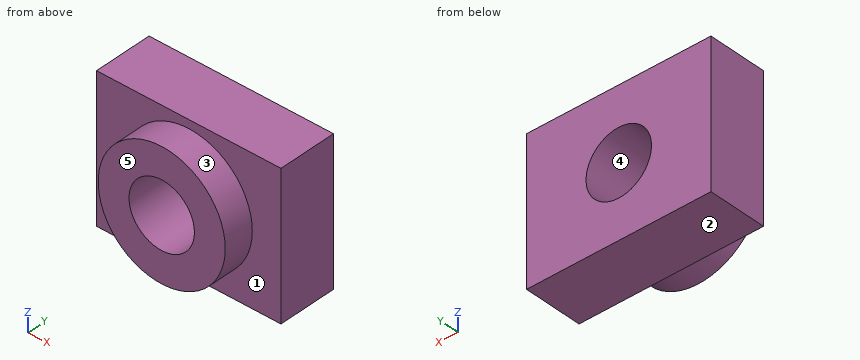
from build123d import *

# Parameters (mm, degrees)
F0_R          = 35.778337
F0_R_2        = 18.424751
F1_DEPTH      = 25
F1_DEPTH_BACK = 25
F0_W          = 103.87025
F0_H          = 80.97905
F2_DEPTH      = 8
F2_DEPTH_BACK = 25


with BuildPart() as f1:
    # F0 (on Front) → F1 (new body, two sides)
    with BuildSketch(Plane.XZ) as f1_sk:
        Circle(F0_R)
        Circle(F0_R_2, mode=Mode.SUBTRACT)
    extrude(amount=F1_DEPTH)
    extrude(f1_sk.sketch, amount=-F1_DEPTH_BACK)

    # F0 (on Front) → F2 (join, two sides)
    with BuildSketch(Plane.XZ) as f2_sk:
        Rectangle(F0_W, F0_H)
        Circle(F0_R, mode=Mode.SUBTRACT)
    extrude(amount=F2_DEPTH)
    extrude(f2_sk.sketch, amount=-F2_DEPTH_BACK)


solid = f1.part
The listing builds one solid part. Answer for the finished solid, in the listing's coordinates (mm). Face numbers are marked on the shaded views. A direction names the side the tool comes from. Round coordinates to 2 decimals unless told otherwise and drop trailing zeros. Write each loop counter-clockwise with the first axis right and the second up, starting at its lowest first coordinate (ties: lowest second). Pieces come first, ordered by that corner, then holes. Notation, with made-up numbers: (61, 3.25) - (82, 3.25) arc R22 cw to (82, 27.25) - close; hole circle Ø8 at (34, 66.5). An arc over 180 degrees is marked (long way). Use one line per item in the form item = value. Start each with the question number.
Item 1: A cutting plane is placed at A-A (z = 0). Write down the section's boundary in (x, y).
Item 2: Determine the mould class of the marked faces 3, 4 and 5 for opening direction Z: +Z half, -Z half, draft (parallel to the pull), parting line (faces both ways), or undercut.
Item 3: Find the intervals of material crossed by line 1 (Z direction, x = 0, y = -12); line 2 (Z direction, x = 0, y = 7); line 3 (Y direction, x = -33.5, z = 29), in increasing order. Write a range as [from, to].
Item 4: A cutting plane is placed at B-B (x = 0). Write down the section's boundary in (y, z), plus the area to 3 significant figures.
Item 5: A cutting plane is placed at C-C (y = -5). Write down the section's boundary in (x, z), plus the area to 3 significant figures.
Item 6: Flat-ended cylindrical pins translate along their axes: pin 1 Ø4 at (y, z) = (-19, 15) entering from +X; pin 2 Ø8 at (y, z) = (-13.5, 27.5) entering from -X; pin 3 Ø3 at (x, z) = (-11, 14.5) entering from +Y; pin 4 Ø2 at (x, z) = (-37, -4.5) entering from -Y. Find the tip coordinate at first contact, or state that the pin passes through.
Item 7: A cutting plane is placed at D-D (z = -26). Write down the section's boundary in (x, y), plus the area to 3 significant figures.
Item 8: A tool of negligible diameter and unlimited length cuts with its end or side. For the marked faces 1 and 2, from which of +Z, -Z, +X, -X, +Y, -Y can it reach the whole face along a straight path? Write none if from no direction.
The answers:
q1.outline = (-51.94, -8) - (-35.78, -8) - (-35.78, -25) - (-18.42, -25) - (-18.42, 25) - (-51.94, 25) - close; (18.42, -25) - (35.78, -25) - (35.78, -8) - (51.94, -8) - (51.94, 25) - (18.42, 25) - close
q2.face_3 = parting line
q2.face_4 = undercut
q2.face_5 = draft
q3.line_1 = [-35.78, -18.42], [18.42, 35.78]
q3.line_2 = [-40.49, -18.42], [18.42, 40.49]
q3.line_3 = [-8, 25]
q4.outline = (-25, -35.78) - (-8, -35.78) - (-8, -40.49) - (25, -40.49) - (25, -18.42) - (-25, -18.42) - close; (-25, 18.42) - (25, 18.42) - (25, 40.49) - (-8, 40.49) - (-8, 35.78) - (-25, 35.78) - close
q4.area = 2,050 mm^2
q5.outline = (-51.94, -40.49) - (51.94, -40.49) - (51.94, 40.49) - (-51.94, 40.49) - close; hole circle Ø36.85 at (0, 0)
q5.area = 7,340 mm^2
q6.pin_1 = 33.33
q6.pin_2 = -26.98
q6.pin_3 = 25
q6.pin_4 = -8
q7.outline = (-51.94, -8) - (-24.58, -8) - (-24.58, -25) - (24.58, -25) - (24.58, -8) - (51.94, -8) - (51.94, 25) - (-51.94, 25) - close
q7.area = 4,260 mm^2
q8.face_1 = -Y
q8.face_2 = -Z, +X, -X, +Y, -Y
